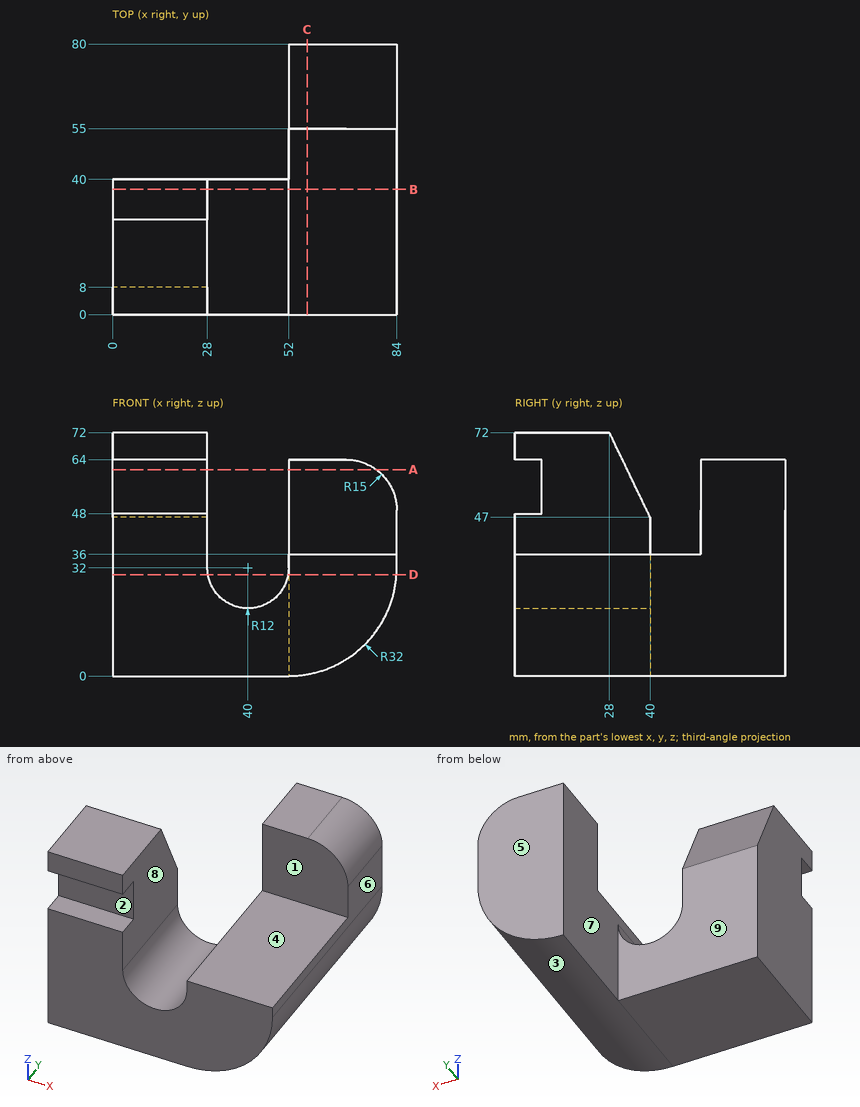
The figure shows three views and two pictorial views of one solid part (mm, origin at its lowest corner). Answer the questions. A direction names the side the tool comes from. Round coordinates to 2 decimals unless told otherwise and drop trailing zeros. Write each loop counter-clockwise with the first axis right and the second up, starting at its lowest first coordinate (ties: lowest second). Pieces come first, ordered by that corner, then holes. Notation, with made-up numbers: (-14.5, -23.5) -> (-2.5, -23.5) arc R25 cw to (-2.5, -6.5) -> close; hole circle Ø10 at (3, -7). An arc over 180 degrees is marked (long way). Write each question's results on one line, items separated by ' | '.
Q1. Determine the mould class of the marked faces 1, 2, 3 and 4 for opening direction Z: released by +Z, released by -Z, zero draft, split by the parting line, or undercut.
Data:
face 1: zero draft | face 2: undercut | face 3: released by -Z | face 4: released by +Z
Q2. Section C-C, the plane x = 57.5 is taken. Write down the section's boundary in (y, z), then the cut area to 3 significant figures.
Data:
outline: (0, 0.48) -> (80, 0.48) -> (80, 64) -> (55, 64) -> (55, 36) -> (0, 36) -> close | area: 3,540 mm^2
Q3. Flat-ended cylindrical pins translate along their axes: P1, Ø1.5, axis at y = 46.5, z = 29, coming from the +X side; P2, Ø3, axis at y = 65, z = 62.5, coming from the -X side; P3, Ø16, axis at x = 69, y = 18.5, coming from the +Z side. Find the tip coordinate at first contact, or state that the pin passes through.
Data:
P1: x = 83.92 | P2: x = 52 | P3: z = 36
Q4. Section A-A, the plane z = 61 is taken. Write down the section's boundary in (x, y).
Data:
outline: (0, 8) -> (28, 8) -> (28, 33.28) -> (0, 33.28) -> close; (52, 55) -> (78, 55) -> (78, 80) -> (52, 80) -> close
Q5. Straight lines are drawn through the part: line 1 along Z through (x, y) = (26, 7); line 2 along X through (y, z) = (10, 35.5); line 3 along X through (y, z) = (21.5, 52.5). For each, find the intervals that lie inside material, in ascending order. Write a range as [from, to].
Data:
line 1: [0, 48], [64, 72] | line 2: [0, 28], [52, 84] | line 3: [0, 28]
Q6. Section D-D, the plane z = 30 is taken. Write down the section's boundary in (x, y).
Data:
outline: (0, 0) -> (28.17, 0) -> (28.17, 40) -> (0, 40) -> close; (51.83, 0) -> (83.94, 0) -> (83.94, 80) -> (52, 80) -> (52, 40) -> (51.83, 40) -> close
Q7. Which of the six approach directions +Z, -Z, +X, -X, +Y, -Y give full straight-line access (tool end or side, diameter ignored) to the marked faces 5, 6, 7, 8 and 9?
Data:
face 5: +Z, -Z, +X, -X, +Y | face 6: +Z, -Z, +X, +Y, -Y | face 7: +Z, +Y | face 8: +Z, +Y, -Y | face 9: +Z, -Z, -X, +Y
Q8. Section B-B, the plane y = 37 is taken. Write down the section's boundary in (x, z).
Data:
outline: (0, 0) -> (52, 0) arc R32 ccw to (84, 32) -> (84, 36) -> (52, 36) -> (52, 32) arc R12 cw to (28, 32) -> (28, 53.25) -> (0, 53.25) -> close
